from build123d import *

# Parameters (mm, degrees)
SKETCH1_R           = 2.5
SKETCH1_R_2         = 4
BOSS_EXTRUDE1_DEPTH = 5


with BuildPart() as part:
    # Sketch1 → Boss-Extrude1 (new body)
    with BuildSketch(Plane.XY):
        with BuildLine():
            Line((-9.688536745, 40), (10.311463255, 40))
            ThreePointArc((10.311463255, 40), (17.382531067, 37.071067812), (20.311463255, 30))
            Line((20.311463255, 30), (20.311463255, -30))
            ThreePointArc((20.311463255, -30), (17.382531067, -37.071067812), (10.311463255, -40))
            Line((10.311463255, -40), (-9.688536745, -40))
            ThreePointArc((-9.688536745, -40), (-16.759604557, -37.071067812), (-19.688536745, -30))
            Line((-19.688536745, -30), (-19.688536745, 30))
            ThreePointArc((-19.688536745, 30), (-16.759604557, 37.071067812), (-9.688536745, 40))
        make_face()
        with Locations((0, 7)):
            Circle(SKETCH1_R, mode=Mode.SUBTRACT)
        with Locations((0, -7)):
            Circle(SKETCH1_R, mode=Mode.SUBTRACT)
        with Locations((-9.688536745, 30)):
            Circle(SKETCH1_R_2, mode=Mode.SUBTRACT)
        with Locations((10.311463255, 30)):
            Circle(SKETCH1_R_2, mode=Mode.SUBTRACT)
        with Locations((-9.688536745, -30)):
            Circle(SKETCH1_R_2, mode=Mode.SUBTRACT)
        with Locations((10.311463255, -30)):
            Circle(SKETCH1_R_2, mode=Mode.SUBTRACT)
        with Locations((-12.688536745, 0)):
            Circle(SKETCH1_R_2, mode=Mode.SUBTRACT)
        with Locations((13.311463255, 0)):
            Circle(SKETCH1_R_2, mode=Mode.SUBTRACT)
        with Locations((-9.688536745, -18)):
            Circle(SKETCH1_R_2, mode=Mode.SUBTRACT)
        with Locations((10.311463255, -18)):
            Circle(SKETCH1_R_2, mode=Mode.SUBTRACT)
        with Locations((10.311463255, 18)):
            Circle(SKETCH1_R_2, mode=Mode.SUBTRACT)
        with Locations((-9.688536745, 18)):
            Circle(SKETCH1_R_2, mode=Mode.SUBTRACT)
    extrude(amount=BOSS_EXTRUDE1_DEPTH)


solid = part.part
Input: part model. Units: mm. Frame: model coordinates. Round coordinates to 2 decimals unless told otherwise and drop trailing zeros. Order: outer loops, then holes, each group sorted by start corner. A loop starts at its lowest first (then second) coordinate and runs counter-clockwise, first axis right, second up. Notation, with made-up numbers: (59.5, -29.5) - (88.5, -29.5) arc R19 ccw to (88.5, -18.5) - close; hole circle Ø4 at (-6.75, -36.5). An arc over 180 degrees is marked (long way). Answer as a JSON object with one key per item and string values. Group by question number.
(1) Cut plane B-B (z = 3.7). Count the separate pieces of the cut face and the enclosed holes in it, then the cut area to 3 significant figures.
(2) Draft query along X for faces 1 (the face through (1, 1, 0)), 2 (the face through (-16.68, -37.15, 2.46)), 3 (the face through (14.127, -16.799, 2.465)). Return one class per face: released by +X, released by -X, zero draft, split by the parting line, or undercut.
(3) Cut plane D-D (x = -10.5). Return loops of the section in (y, z), then the cut area to 3 significant figures.
(4) Pin query (flat end, axial travel): P1, Ø3, axis at x = 0, y = 7, coming from the +Z side; P2, Ø9, axis at x = 10.31, y = 30, coming from the +Z side. Return the tip coordinate at first contact, or that it passes through.
(5) Material intervals for probe 1 along Y at (x, z) = (0, 1.25); probe 2 along Y at (x, z) = (12.5, 3.45); probe 3 along Y at (x, z) = (8.5, 3.4), sorted ascending. Write a range as from..to.
(6) Cut plane A-A (y = -18). Return loops of the section in (x, z), then the cut area to 3 significant figures.
(7) Cut plane C-C (y = 7). Return loops of the section in (x, z), then the cut area to 3 significant figures.
Here are the results:
{
 "1": {"separate pieces": "1", "enclosed holes": "12", "area": "2,570 mm^2"},
 "2": {"face 1": "zero draft", "face 2": "released by -X", "face 3": "undercut"},
 "3": {"outline": "(-39.97, 0) - (-33.92, 0) - (-33.92, 5) - (-39.97, 5) - close; (-26.08, 0) - (-21.92, 0) - (-21.92, 5) - (-26.08, 5) - close; (-14.08, 0) - (-3.35, 0) - (-3.35, 5) - (-14.08, 5) - close; (3.35, 0) - (14.08, 0) - (14.08, 5) - (3.35, 5) - close; (21.92, 0) - (26.08, 0) - (26.08, 5) - (21.92, 5) - close; (33.92, 0) - (39.97, 0) - (39.97, 5) - (33.92, 5) - close", "area": "210 mm^2"},
 "4": {"P1": "passes through", "P2": "stops at z = 5"},
 "5": {"probe 1": "y = -40..-9.5, -4.5..4.5, 9.5..40", "probe 2": "y = -39.76..-33.35, -26.65..-21.35, -14.65..-3.92, 3.92..14.65, 21.35..26.65, 33.35..39.76", "probe 3": "y = -40..-33.57, -26.43..-21.57, -14.43..14.43, 21.57..26.43, 33.57..40"},
 "6": {"outline": "(-19.69, 0) - (-13.69, 0) - (-13.69, 5) - (-19.69, 5) - close; (-5.69, 0) - (6.31, 0) - (6.31, 5) - (-5.69, 5) - close; (14.31, 0) - (20.31, 0) - (20.31, 5) - (14.31, 5) - close", "area": "120 mm^2"},
 "7": {"outline": "(-19.69, 0) - (-2.5, 0) - (-2.5, 5) - (-19.69, 5) - close; (2.5, 0) - (20.31, 0) - (20.31, 5) - (2.5, 5) - close", "area": "175 mm^2"}
}
